from build123d import *

# Parameters (mm, degrees)
SKETCH007_R         = 15
EXTRUDE003004_DEPTH = 0.4
BOX019_W            = 17
BOX019_H            = 0.4
BOX019_DEPTH        = 20
BOX018_W            = 17
BOX018_H            = 4.35
BOX018_DEPTH        = 28
BOX013_W            = 1
BOX013_H            = 5.2
BOX013_DEPTH        = 3
CYLINDER009_R       = 4.15
CYLINDER009_DEPTH   = 10
CYLINDER007_R       = 4.15
CYLINDER007_DEPTH   = 10
BOX007_W            = 50
BOX007_H            = 25
BOX007_DEPTH        = 0.5
SKETCH006_R         = 15
EXTRUDE003003_DEPTH = 17.25


with BuildPart() as extrude003004:
    # Sketch007 → Extrude003004 (new body)
    with BuildSketch(Plane.XZ):
        with Locations((89, 10.4)):
            Circle(SKETCH007_R)
    extrude(amount=EXTRUDE003004_DEPTH)


with BuildPart() as extrude003004_1:
    # Extrude003004 placement: moved
    add(extrude003004.part.moved(Location((0, -17, 0))))


with BuildPart() as cube016:
    # Box019 → Box019 (new body)
    with BuildSketch(Plane(origin=(80.5, -17.3, 2), x_dir=(1, 0, 0), z_dir=(0, 0, 1))):
        with Locations((8.5, 0.2)):
            Rectangle(BOX019_W, BOX019_H)
    extrude(amount=BOX019_DEPTH)


with BuildPart() as cube015:
    # Box018 → Box018 (new body)
    with BuildSketch(Plane(origin=(80.5, -17.3, 10), x_dir=(1, 0, 0), z_dir=(0, 0, 1))):
        with Locations((8.5, 2.175)):
            Rectangle(BOX018_W, BOX018_H)
    extrude(amount=BOX018_DEPTH)


with BuildPart() as cube012:
    # Box013 → Box013 (new body)
    with BuildSketch(Plane(origin=(88.5, -18.1, 9), x_dir=(1, 0, 0), z_dir=(0, 0, 1))):
        with Locations((0.5, 2.6)):
            Rectangle(BOX013_W, BOX013_H)
    extrude(amount=BOX013_DEPTH)


with BuildPart() as obj1:
    # Cylinder009 → Cylinder009 (new body)
    with BuildSketch(Plane(origin=(93.2, -12.9, 10.4), x_dir=(1, 0, 0), z_dir=(0, -1, 0))):
        Circle(CYLINDER009_R)
    extrude(amount=CYLINDER009_DEPTH)


with BuildPart() as obj2:
    # Cylinder007 → Cylinder007 (new body)
    with BuildSketch(Plane(origin=(84.8, -12.9, 10.4), x_dir=(1, 0, 0), z_dir=(0, -1, 0))):
        Circle(CYLINDER007_R)
    extrude(amount=CYLINDER007_DEPTH)


with BuildPart() as cube007:
    # Box007 → Box007 (new body)
    with BuildSketch(Plane(origin=(66, 0, -2), x_dir=(1, 0, 0), z_dir=(0, -1, 0))):
        with Locations((25, 12.5)):
            Rectangle(BOX007_W, BOX007_H)
    extrude(amount=BOX007_DEPTH)


with BuildPart() as obj3:
    # Sketch006 → Extrude003003 (new body)
    with BuildSketch(Plane.XZ):
        with Locations((89, 10.4)):
            Circle(SKETCH006_R)
    extrude(amount=EXTRUDE003003_DEPTH)

    # Cut005014006: cut Cube007
    add(cube007.part, mode=Mode.SUBTRACT)

    # Cut005014007: cut obj2
    add(obj2.part, mode=Mode.SUBTRACT)

    # Cut005014010: cut obj1
    add(obj1.part, mode=Mode.SUBTRACT)

    # Cut005014011: cut Cube012
    add(cube012.part, mode=Mode.SUBTRACT)

    # Cut005014013: cut Cube015
    add(cube015.part, mode=Mode.SUBTRACT)

    # Fusion007: union Cube016
    add(cube016.part)

    # Fusion008: union Extrude003004
    add(extrude003004_1.part)


solid = obj3.part
Build history of the part. All positions in model axes, mm. A direction names the side the tool comes from. Round coordinates to 2 decimals unless told otherwise and drop trailing zeros. Write each loop counter-clockwise with the first axis right and the second up, starting at its lowest first coordinate (ties: lowest second). Pieces come first, ordered by that corner, then holes. Notation, with made-up numbers: (10, -5) - (32, -5) arc R19 cw to (32, 26) - close; hole circle Ø5 at (28, -14.5). An arc over 180 degrees is marked (long way). Use CSV: the item, a comma, the result in double quotes.
(1) Band-saw the part on C-C (y = -10.25). Write the cut outline in (x, z), plus the area to 3 significant figures.
Response:
outline,"circle Ø30 at (89, 10.4)"
area,"707 mm²"
(2) Mould opens along X. For faces 1 (the flat face through (89, 0, -3)), 2 (the flat face through (80.5, -15, 16)), 3 (the cylindrical face through (85.748, -8.578, -4.243)) say: pulls with the +X half, pulls with the -X half, needs draft (parallel to the pull), parting line crosses it, or undercut.
Response:
face 1,"needs draft"
face 2,"undercut"
face 3,"parting line crosses it"
(3) 3-axis set-ups, long thin cutter, end or side, ignore diameter. For faces 4 (the flat face through (89, -12.9, 10)), 5 (the flat face through (89, -16.9, 14)), 6 (the flat face through (89, -0.5, 11)): which of +Z, -Z, +X, -X, +Y, -Y reach the whole face in a straight line?
Response:
face 4,"none"
face 5,"+Z"
face 6,"+X, -X, +Y"
(4) Pin check, flat tips, straight feed: P1, Ø8, axis at y = -5, z = 21.5, coming from the +X side; P2, Ø5, axis at y = -9.5, z = 6, coming from the +X side; P3, Ø6, axis at y = -2, z = 9.5, coming from the -X side; P4, Ø0.6, axis at x = 91.5, y = 0, coming from the -Z side. Stop position of each tip, or through.
Response:
P1,"x = 102.21"
P2,"x = 103.88"
P3,"x = 74"
P4,"z = -4.44"
(5) Band-saw the part on B-B (z = 10.4). Write the cut outline in (x, y), plus the area to 3 significant figures.
Response:
outline,"(74, -17.4) - (104, -17.4) - (104, -0.5) - (74, -0.5) - close; hole (80.5, -16.9) - (97.5, -16.9) - (97.5, -12.95) - (97.35, -12.95) - (97.35, -12.9) - (80.65, -12.9) - (80.65, -12.95) - (80.5, -12.95) - close"
area,"439 mm²"
(6) Wall check: line 1 (X direction, y = -14.9, z = 10.4); line 2 (Y direction, x = 91.25, z = 16); line 3 (X direction, y = -15, z = 7.75). Give the ranges that are in metal, low to high.
Response:
line 1,"74 to 80.5, 97.5 to 104"
line 2,"-17.4 to -16.9, -12.95 to -0.5"
line 3,"74.24 to 81.61, 87.99 to 90.01, 96.39 to 103.76"
(7) Band-saw the part on A-A (x = 84.8). Write the cut outline in (y, z).
Response:
outline,"(-17.4, -4) - (0, -4) - (0, -2) - (-0.5, -2) - (-0.5, 23) - (0, 23) - (0, 24.8) - (-12.95, 24.8) - (-12.95, 14.55) - (-12.9, 14.55) - (-12.9, 6.25) - (-16.9, 6.25) - (-16.9, 22) - (-17, 22) - (-17, 24.8) - (-17.4, 24.8) - close"
